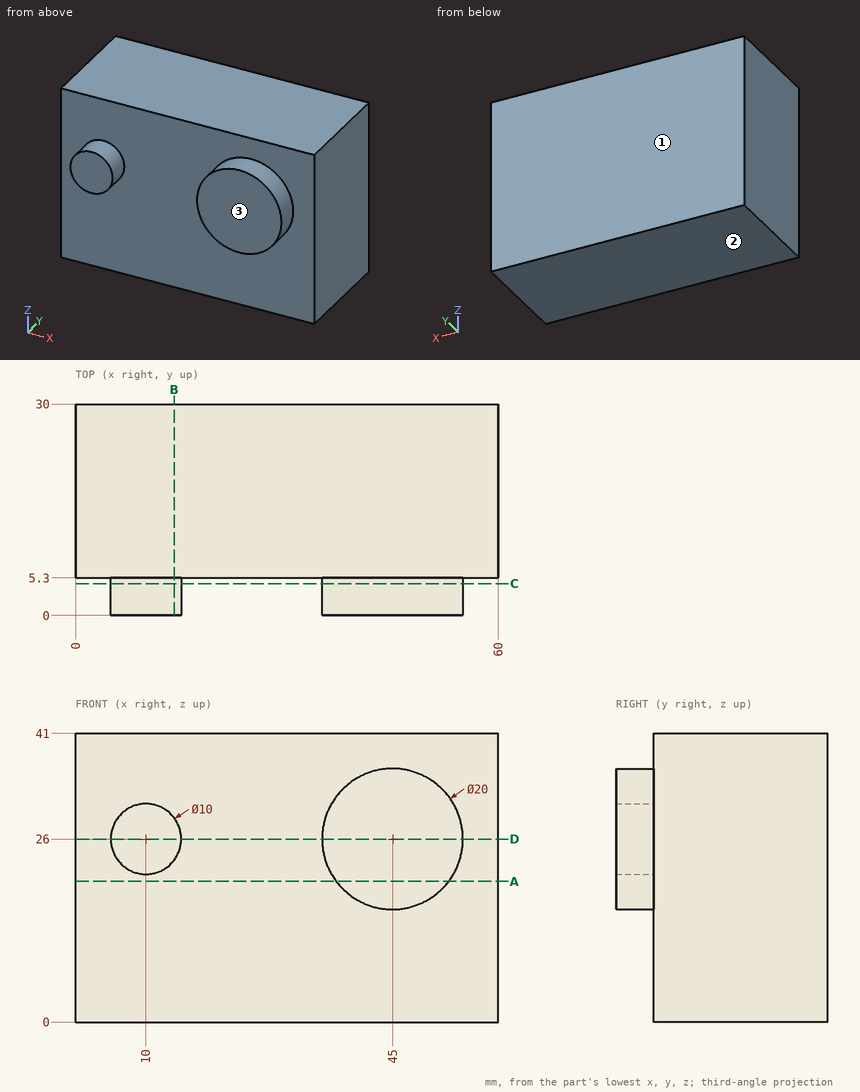
The figure shows three views and two pictorial views of one solid part (mm, origin at its lowest corner). Answer the questions. Coordinates: 2 decimals unless noted, no trailing zeros. Loops run counter-clockwise (first coordinate to the right, second up) from the corner with the lowest first, then second, coordinate; pieces in that order, holes last. Notation, with made-up numbers: M 40.5,-7.75 L 77.5,-7.75 A4 cw 77.5,-0.75 Z; hole C -39.75,21 d10. An arc over 180 degrees is marked long. Use CSV: the item, a comma, the result in double quotes. Start each with the question number.
(1) Find section A-A, the plane z = 20. Give the vertices of the cut face in (x, y), then the cut area to 3 significant figures.
(2) Find section C-C, the plane y = 4.5. Give the vertices of the cut face in (x, z), then the cut area to 3 significant figures.
(3) Consider line 1 (Y direction, x = 19.5, z = 16.5); line 2 (Z direction, x = 42.5, y = 5); line 3 (Z direction, x = 9, y = 2.25). Determine where each line is inside the solid, lowest interval first.
(4) Find section D-D, the plane z = 26. Give the vertices of the cut face in (x, y).
(5) Given pin 1 Ø1.5 at (x, z) = (12, 18.5) entering from -Y, flat-ended and moving along its own axis, determine where the tip first touches the part or whether it passes through.
(6) Find section B-B, the plane x = 14. Give the vertices of the cut face in (y, z), then the cut area to 3 significant figures.
(7) For a pull along Y with two mould halves and no side action, classify the marked faces 1, 2 and 3 as +Y half, -Y half, draft (parallel to the pull), parting line (faces both ways), or undercut.
Recorded:
1,outline,"M 0,5.3 L 37,5.3 L 37,0 L 53,0 L 53,5.3 L 60,5.3 L 60,30 L 0,30 Z"
1,area,"1,570 mm^2"
2,outline,"C 10,26 d10; C 45,26 d20"
2,area,"393 mm^2"
3,line 1,"y = 5.3 to 30"
3,line 2,"z = 16.32 to 35.68"
3,line 3,"z = 21.1 to 30.9"
4,outline,"M 0,5.3 L 5,5.3 L 5,0 L 15,0 L 15,5.3 L 35,5.3 L 35,0 L 55,0 L 55,5.3 L 60,5.3 L 60,30 L 0,30 Z"
5,pin 1,"stops at y = 5.3"
6,outline,"M 0,23 L 5.3,23 L 5.3,0 L 30,0 L 30,41 L 5.3,41 L 5.3,29 L 0,29 Z"
6,area,"1,040 mm^2"
7,face 1,"+Y half"
7,face 2,"draft"
7,face 3,"-Y half"
